from build123d import *

# Parameters (mm, degrees)
F0_R     = 30
F1_DEPTH = 75
F2_R     = 20
F3_DEPTH = 75
F4_R     = 59.37587
F5_DEPTH = 25


with BuildPart() as f1:
    # F0 (on Top) → F1 (new body)
    with BuildSketch(Plane.XY):
        Circle(F0_R)
    extrude(amount=F1_DEPTH)

    # F2 (on Top) → F3 (cut, through all)
    with BuildSketch(Plane.XY):
        Circle(F2_R)
    extrude(amount=F3_DEPTH, mode=Mode.SUBTRACT)

    # F4 (on Top) → F5 (join)
    with BuildSketch(Plane.XY):
        Circle(F4_R)
    extrude(amount=F5_DEPTH)


solid = f1.part
Source: CAD feature listing. Evaluate the final solid. Frame: model axes, mm. A direction names the side the tool comes from. Coordinates: 2 decimals unless noted, no trailing zeros. Loops run counter-clockwise (first coordinate to the right, second up) from the corner with the lowest first, then second, coordinate; pieces in that order, holes last. Notation, with made-up numbers: M -28.5,31.25 L 11.5,31.25 A23 cw 11.5,39.25 Z; hole C 6.25,-29 d6. An arc over 180 degrees is marked long. Answer in a Markdown table with one row per item.
Q1. Section A-A on y = 0. Return the cut outline in (x, z).
Answers below:
| item | result |
|---|---|
| outline | M -59.38,0 L 59.38,0 L 59.38,25 L 30,25 L 30,75 L 20,75 L 20,25 L -20,25 L -20,75 L -30,75 L -30,25 L -59.38,25 Z |
Q2. Section D-D on z = 19.5. Return the cut outline in (x, y), plus the area to 3 significant figures.
Answers below:
| item | result |
|---|---|
| outline | C 0,0 d118.75 |
| area | 11,100 mm^2 |
Q3. Section C-C on z = 31.5. Return the cut outline in (x, y), plus the area to 3 significant figures.
Answers below:
| item | result |
|---|---|
| outline | C 0,0 d60; hole C 0,0 d40 |
| area | 1,570 mm^2 |
Q4. Ray query, probe 1 along Y at (x, z) = (0, 45); probe 2 along Z at (x, y) = (-42, -33.5). Return the intervals inside material, ascending. Write a range as from..to.
Answers below:
| item | result |
|---|---|
| probe 1 | y = -30..-20, 20..30 |
| probe 2 | z = 0..25 |
Q5. Set-up query: faces 1 (the flat face through (-27, 14, 25)), 2 (the flat face through (-1, 1, 0)). Return all of +Z, -Z, +X, -X, +Y, -Y with unobstructed straight access to the full face (end or side cutting, diameter ignored); none if empty.
Answers below:
| item | result |
|---|---|
| face 1 | +Z |
| face 2 | -Z, +X, -X, +Y, -Y |
Q6. First-contact query: pin 1 (10 mm diameter, centred on y = 24, z = 56.5, fed in from +X); pin 2 (24 mm diameter, centred on x = 0, y = 0, fed in from +Z); pin 3 (12 mm diameter, centred on x = 40.5, z = 64.5, fed in from +Y); pin 4 (8 mm diameter, centred on x = 18.5, z = 67, fed in from +Y). Flat tips, straight axial feed; report the tip coordinate or a pass-through.
Answers below:
| item | result |
|---|---|
| pin 1 | stops at x = 23.22 |
| pin 2 | stops at z = 25 |
| pin 3 | passes through |
| pin 4 | stops at y = 26.26 |
